Could you check a few things on this model? Use its own coordinates, in mm. A direction names the side the tool comes from. Round coordinates to 2 decimals unless told otherwise and drop trailing zeros. Write each loop counter-clockwise with the first axis right and the second up, starting at its lowest first coordinate (ties: lowest second). Pieces come first, ordered by that corner, then holes. Notation, with made-up numbers: (73, 72) -> (84, 72) arc R24 ccw to (84, 94) -> close; hole circle Ø7 at (8.25, 13). An arc over 180 degrees is marked (long way). Answer in a Markdown table with one row per item.
from build123d import *

# Parameters (mm, degrees)
SKETCH2_W           = 64
SKETCH2_H           = 58.3
BOSS_EXTRUDE1_DEPTH = 5
SKETCH3_R           = 2.5
CUT_EXTRUDE1_DEPTH  = 10
FILLET1_R           = 5
SKETCH4_R           = 12.5
CUT_EXTRUDE2_DEPTH  = 10


with BuildPart() as part:
    # Sketch2 → Boss-Extrude1 (new, symmetric)
    with BuildSketch(Plane.XY):
        Rectangle(SKETCH2_W, SKETCH2_H)
        with BuildLine():
            ThreePointArc((-25.125, 23.85), (-21.875, 27.1), (-18.625, 23.85))
            Line((-18.625, 23.85), (-18.625, 13.85))
            ThreePointArc((-18.625, 13.85), (-21.875, 10.6), (-25.125, 13.85))
            Line((-25.125, 13.85), (-25.125, 23.85))
        make_face(mode=Mode.SUBTRACT)
        with BuildLine():
            Line((18.625, 13.85), (18.625, 23.85))
            ThreePointArc((18.625, 23.85), (21.875, 27.1), (25.125, 23.85))
            Line((25.125, 23.85), (25.125, 13.85))
            ThreePointArc((25.125, 13.85), (21.875, 10.6), (18.625, 13.85))
        make_face(mode=Mode.SUBTRACT)
    extrude(amount=BOSS_EXTRUDE1_DEPTH, both=True)

    # Sketch3 → Cut-Extrude1 (cut)
    with BuildSketch(Plane.XZ.offset(29.15)):
        with Locations(Location((-24, 0, 0), (0, 0, 270))):
            Circle(SKETCH3_R)
        with Locations(Location((24, 0, 0), (0, 0, 90))):
            Circle(SKETCH3_R)
    extrude(amount=-CUT_EXTRUDE1_DEPTH, mode=Mode.SUBTRACT)

    # Fillet1
    fillet1_edges = [part.edges().sort_by_distance(p)[0] for p in [
        (-32, 29.15, 0),
        (32, 29.15, 0),
    ]]
    fillet(fillet1_edges, radius=FILLET1_R)

    # Sketch4 → Cut-Extrude2 (cut)
    with BuildSketch(Plane.XY.offset(5)):
        Circle(SKETCH4_R)
    extrude(amount=-CUT_EXTRUDE2_DEPTH, mode=Mode.SUBTRACT)


solid = part.part
1) Thinking about a two-plate mould opening in X: for faces 1 (the face through (-24, -19.15, 0)), 2 (the face through (32, -3, 0)), 3 (the face through (0, -29.15, 0)), 4 (the face through (-32, -3, 0)), which applies, +X half, -X half, draft (parallel to the pull), parting line (faces both ways), or undercut?
Findings:
| item | result |
|---|---|
| face 1 | undercut |
| face 2 | +X half |
| face 3 | draft |
| face 4 | -X half |
2) For faces 5 (the face through (-21.8, 10.6, 0.1)), 6 (the face through (21.52, -24.22, -0.33)), 7 (the face through (0, -13, -5)), which set-ups out of +Z, -Z, +X, -X, +Y, -Y let a thin tool reach every point of the face, with its end or its side?
Findings:
| item | result |
|---|---|
| face 5 | +Z, -Z |
| face 6 | -Y |
| face 7 | -Z, +X, -X, +Y, -Y |
3) Please list where these lines run through material, in increasing order: line 1 (X direction, y = -22.5, z = 0); line 2 (Y direction, x = 0, z = -0.75); line 3 (Z direction, x = 24, y = -21).
Findings:
| item | result |
|---|---|
| line 1 | x = -32 to -26.5, -21.5 to 21.5, 26.5 to 32 |
| line 2 | y = -29.15 to -12.5, 12.5 to 29.15 |
| line 3 | z = -5 to -2.5, 2.5 to 5 |
4) Imagine slicing it at C-C, the plane z = -0.75. Please give me the cut outline in (x, y) (3 decimals), plus the area to 3 significant figures.
Findings:
| item | result |
|---|---|
| outline | (-32, -29.15) -> (-26.385, -29.15) -> (-26.385, -19.15) -> (-21.615, -19.15) -> (-21.615, -29.15) -> (21.615, -29.15) -> (21.615, -19.15) -> (26.385, -19.15) -> (26.385, -29.15) -> (32, -29.15) -> (32, 24.15) arc R5 ccw to (27, 29.15) -> (-27, 29.15) arc R5 ccw to (-32, 24.15) -> close; hole (-25.125, 13.85) arc R3.25 ccw to (-18.625, 13.85) -> (-18.625, 23.85) arc R3.25 ccw to (-25.125, 23.85) -> close; hole circle Ø25 at (0, 0); hole (18.625, 13.85) arc R3.25 ccw to (25.125, 13.85) -> (25.125, 23.85) arc R3.25 ccw to (18.625, 23.85) -> close |
| area | 2,940 mm^2 |
5) Imagine slicing it at D-D, the plane y = -21. Please give me the cut outline in (x, z).
Findings:
| item | result |
|---|---|
| outline | (-32, -5) -> (32, -5) -> (32, 5) -> (-32, 5) -> close; hole circle Ø5 at (-24, 0); hole circle Ø5 at (24, 0) |
6) Imagine slicing it at B-B, the plane y = 8. Please give me the cut outline in (x, z), plus the area to 3 significant figures.
Findings:
| item | result |
|---|---|
| outline | (-32, -5) -> (-9.6, -5) -> (-9.6, 5) -> (-32, 5) -> close; (9.6, -5) -> (32, -5) -> (32, 5) -> (9.6, 5) -> close |
| area | 448 mm^2 |
7) Imagine slicing it at A-A, the plane x = 0. Please give me the cut outline in (y, z), plus the area to 3 significant figures.
Findings:
| item | result |
|---|---|
| outline | (-29.15, -5) -> (-12.5, -5) -> (-12.5, 5) -> (-29.15, 5) -> close; (12.5, -5) -> (29.15, -5) -> (29.15, 5) -> (12.5, 5) -> close |
| area | 333 mm^2 |
8) For pin 1 (1.5 mm diameter, centred on x = -23.5, z = -0.5, fed in from -Y), with a flat end and sliding along its axis, tell me the tip position at first contact or that it passes through.
Findings:
| item | result |
|---|---|
| pin 1 | stops at y = -19.15 |
